from build123d import *

# Parameters (mm, degrees)
BOSS_EXTRUDE1_DEPTH      = 18
BOSS_EXTRUDE1_DEPTH_BACK = 12.815459
SKETCH1_W                = 72.5
SKETCH1_H                = 96.828401578
SHELL1_T                 = 2
SKETCH2_R                = 7.5
CUT_EXTRUDE1_DEPTH       = 2
CHAMFER1_SIZE            = 1
SKETCH5_R                = 5.5
CUT_EXTRUDE2_DEPTH       = 2
CHAMFER2_SIZE            = 1
SKETCH8_W                = 72.5
SKETCH8_H                = 96.828401578
CUT_EXTRUDE5_DEPTH       = 8
BOSS_EXTRUDE3_START      = 10
SKETCH10_W               = 70.5
SKETCH10_H               = 94.828401578
SKETCH10_W_2             = 68.5
SKETCH10_H_2             = 92.828401578
BOSS_EXTRUDE3_DEPTH      = 2
CUT_EXTRUDE6_REACH       = 183.831
SKETCH12_R               = 1.6
FILLET1_R                = 2
BOSS_EXTRUDE4_START      = 10
SKETCH13_R               = 1.65
BOSS_EXTRUDE4_DEPTH      = 2
SKETCH16_R               = 1.65
BOSS_EXTRUDE5_DEPTH      = 2
SKETCH17_R               = 1.65
CUT_EXTRUDE8_DEPTH       = 12.81545914
SKETCH19_W               = 44.967113154
SKETCH19_H               = 24.357186292
BOSS_EXTRUDE6_DEPTH      = 12
CUT_EXTRUDE9_START       = -10.815459
SKETCH18_R               = 3
CUT_EXTRUDE9_DEPTH       = 14
SKETCH14_R               = 1.599946
CUT_EXTRUDE7_DEPTH       = 2


with BuildPart() as part:
    # Sketch1 → Boss-Extrude1 (new, two sides: drawn at the far end of the back side and taken through both)
    with BuildSketch(Plane(origin=(0, 0, 0), x_dir=(1, 0, 0), z_dir=(0, 1, 0)).offset(-BOSS_EXTRUDE1_DEPTH_BACK)):
        with Locations((117.12025684, -15.018542133)):
            Rectangle(SKETCH1_W, SKETCH1_H)
    extrude(amount=BOSS_EXTRUDE1_DEPTH + BOSS_EXTRUDE1_DEPTH_BACK)

    # Shell1 (no face opened: a closed hollow body)
    add(offset(amount=-SHELL1_T, mode=Mode.PRIVATE), mode=Mode.SUBTRACT)

    # Sketch2 → Cut-Extrude1 (cut)
    with BuildSketch(Plane(origin=(0, 0, -33.395658656), x_dir=(-1, 0, 0), z_dir=(0, 0, -1))):
        with Locations((-114.89374317, -0.00045914)):
            Circle(SKETCH2_R)
    extrude(amount=-CUT_EXTRUDE1_DEPTH, mode=Mode.SUBTRACT)

    # Chamfer1
    chamfer1_edges = [part.edges().sort_by_distance(p)[0] for p in [
        (122.39374317, -0.00045914, -33.395658656),
    ]]
    chamfer(chamfer1_edges, length=CHAMFER1_SIZE)

    # Sketch5 → Cut-Extrude2 (cut)
    with BuildSketch(Plane.XY.offset(63.432742922)):
        with Locations((100.762134065, -2.34045914)):
            Circle(SKETCH5_R)
    extrude(amount=-CUT_EXTRUDE2_DEPTH, mode=Mode.SUBTRACT)

    # Chamfer2
    chamfer2_edges = [part.edges().sort_by_distance(p)[0] for p in [
        (95.262134065, -2.34045914, 63.432742922),
    ]]
    chamfer(chamfer2_edges, length=CHAMFER2_SIZE)

    # Sketch8 → Cut-Extrude5 (cut)
    with BuildSketch(Plane(origin=(0, 18, 0), x_dir=(1, 0, 0), z_dir=(0, 1, 0))):
        with Locations((117.12025684, -15.018542133)):
            Rectangle(SKETCH8_W, SKETCH8_H)
    extrude(amount=-CUT_EXTRUDE5_DEPTH, mode=Mode.SUBTRACT)

    # Sketch10 → Boss-Extrude3 (add)
    with BuildSketch(Plane(origin=(0, 0, 0), x_dir=(1, 0, 0), z_dir=(0, 1, 0)).offset(BOSS_EXTRUDE3_START)):
        with Locations((117.12025684, -15.018542133)):
            Rectangle(SKETCH10_W, SKETCH10_H)
        with Locations((117.12025684, -15.018542133)):
            Rectangle(SKETCH10_W_2, SKETCH10_H_2, mode=Mode.SUBTRACT)
    extrude(amount=BOSS_EXTRUDE3_DEPTH)

    # Sketch12 → Cut-Extrude6 (cut, up to next)
    with BuildSketch(Plane.XY.offset(63.432742922), mode=Mode.PRIVATE) as cut_extrude6_sk1:
        with Locations((109.796270245, -4.680244976)):
            Circle(SKETCH12_R)
    cut_extrude6_tool1 = extrude(cut_extrude6_sk1.sketch, amount=-CUT_EXTRUDE6_REACH, mode=Mode.PRIVATE) & part.part
    add(cut_extrude6_tool1.solids().sort_by_distance((109.79627, -4.680245, 63.432743))[0], mode=Mode.SUBTRACT)

    # Fillet1
    fillet1_edges = [part.edges().sort_by_distance(p)[0] for p in [
        (80.87025684, -1.4077295, -33.395658656),
        (153.37025684, -1.4077295, -33.395658656),
        (153.37025684, -1.4077295, 63.432742922),
        (80.87025684, -1.4077295, 63.432742922),
    ]]
    fillet(fillet1_edges, radius=FILLET1_R)

    # Sketch13 → Boss-Extrude4 (add)
    with BuildSketch(Plane(origin=(0, 0, 0), x_dir=(1, 0, 0), z_dir=(0, 1, 0)).offset(BOSS_EXTRUDE4_START)):
        with BuildLine():
            Line((111.12025684, -63.432742922), (123.12025684, -63.432742922))
            ThreePointArc((123.12025684, -63.432742922), (117.12025684, -69.432742922), (111.12025684, -63.432742922))
        make_face()
        with Locations(Location((117.12025684, -66.432742922, 0), (0, 0, 270))):
            Circle(SKETCH13_R, mode=Mode.SUBTRACT)
    boss_extrude4 = extrude(amount=-BOSS_EXTRUDE4_DEPTH)

    # Sketch16 → Boss-Extrude5 (add)
    with BuildSketch(Plane(origin=(0, 10, 0), x_dir=(1, 0, 0), z_dir=(0, 1, 0))):
        with BuildLine():
            Line((111.12025684, 33.395658656), (123.12025684, 33.395658656))
            ThreePointArc((123.12025684, 33.395658656), (117.12025684, 39.395658656), (111.12025684, 33.395658656))
        make_face()
        with Locations(Location((117.12025684, 36.395658656, 0), (0, 0, 270))):
            Circle(SKETCH16_R, mode=Mode.SUBTRACT)
    extrude(amount=-BOSS_EXTRUDE5_DEPTH)

    # Sketch17 → Cut-Extrude8 (cut)
    with BuildSketch(Plane(origin=(0, 0, 0), x_dir=(1, 0, 0), z_dir=(0, 1, 0))):
        with Locations(Location((137.785174065, -38.462742922, 0), (0, 0, 90))):
            Circle(SKETCH17_R)
        with Locations(Location((89.525174065, -37.192742922, 0), (0, 0, 90))):
            Circle(SKETCH17_R)
    extrude(amount=-CUT_EXTRUDE8_DEPTH, mode=Mode.SUBTRACT)

    # Sketch19 → Boss-Extrude6 (add)
    with BuildSketch(Plane.XZ.offset(12.81545914)):
        with Locations((117.12025684, 15.018542133)):
            Rectangle(SKETCH19_W, SKETCH19_H)
    extrude(amount=BOSS_EXTRUDE6_DEPTH)

    # Sketch18 → Cut-Extrude9 (cut)
    with BuildSketch(Plane(origin=(0, 0, 0), x_dir=(1, 0, 0), z_dir=(0, 1, 0)).offset(CUT_EXTRUDE9_START)):
        with Locations(Location((124.62025684, -15.018542133, 0), (0, 0, 270))):
            Circle(SKETCH18_R)
        with Locations(Location((109.62025684, -15.018542133, 0), (0, 0, 270))):
            Circle(SKETCH18_R)
    extrude(amount=-CUT_EXTRUDE9_DEPTH, mode=Mode.SUBTRACT)

    # Mirror1: Boss-Extrude4 across plane
    add(boss_extrude4.mirror(Plane.XY.offset(15.018542133)))

    # Sketch14 → Cut-Extrude7 (cut)
    with BuildSketch(Plane(origin=(0, -10.81545914, 0), x_dir=(1, 0, 0), z_dir=(0, 1, 0))):
        with Locations(Location((140.517827737, -46.462742922, 0), (0, 0, 270))):
            Circle(SKETCH14_R)
        with Locations(Location((92.257827737, -45.192742922, 0), (0, 0, 270))):
            Circle(SKETCH14_R)
    extrude(amount=-CUT_EXTRUDE7_DEPTH, mode=Mode.SUBTRACT)


solid = part.part
CAD build for the part. Positions are in the model's coordinates, mm. A direction names the side the tool comes from. Coordinates: 2 decimals unless noted, no trailing zeros. Order: outer loops, then holes, each group sorted by start corner. A loop starts at its lowest first (then second) coordinate and runs counter-clockwise, first axis right, second up.
Item 1: Band-saw the part on B-B on z = 29. List the corners of the cut face in (x, y).
Check sheet entries:
outline: (80.87, -12.82) - (153.37, -12.82) - (153.37, 10) - (152.37, 10) - (152.37, 12) - (151.37, 12) - (151.37, -10.82) - (82.87, -10.82) - (82.87, 12) - (81.87, 12) - (81.87, 10) - (80.87, 10) - close
Item 2: Two-plate mould, pull along X, no slides. Class faces 1 (the face through (117, 8, 64)), 2 (the face through (80.87, -2, 16)), 3 (the face through (117, 0, 61.433)): +X half, -X half, draft (parallel to the pull), parting line (faces both ways), or undercut.
Check sheet entries:
face 1: draft
face 2: -X half
face 3: undercut
Item 3: Band-saw the part on A-A on x = 144.5. List the corners of the cut face in (y, z), plus the area to 3 significant figures.
Check sheet entries:
outline: (-12.82, -33.4) - (10, -33.4) - (10, -32.4) - (12, -32.4) - (12, -31.4) - (-10.82, -31.4) - (-10.82, 61.43) - (12, 61.43) - (12, 62.43) - (10, 62.43) - (10, 63.43) - (-12.82, 63.43) - close
area: 281 mm2
Item 4: Pin check, flat tips, straight feed: pin 1 Ø1.5 at (x, z) = (132.5, -10.5) entering from +Y; pin 2 Ø10 at (x, y) = (94.5, 1.5) entering from -Z; pin 3 Ø5 at (x, z) = (126.5, 17) entering from -Y; pin 4 Ø1.6 at (y, z) = (11, -6) entering from +X. Stop position of each tip, or through.
Check sheet entries:
pin 1: stops at y = -10.82
pin 2: stops at z = -33.4
pin 3: stops at y = -24.82
pin 4: stops at x = 152.37
Item 5: Band-saw the part on C-C on y = -18. List the corners of the cut face in (x, z).
Check sheet entries:
outline: (94.64, 2.84) - (139.6, 2.84) - (139.6, 27.2) - (94.64, 27.2) - close; hole circle Ø6 at (109.62, 15.02); hole circle Ø6 at (124.62, 15.02)
Item 6: 3-axis set-ups, long thin cutter, end or side, ignore diameter. For faces 4 (the face through (108.2, -4.6, 62.4)), 5 (the face through (136.15, -11.8, 38.68)), 6 (the face through (151.37, 0, 16)), 7 (the face through (117, -19, 27.197)): which of +Z, -Z, +X, -X, +Y, -Y reach the whole face in a straight line?
Check sheet entries:
face 4: +Z
face 5: +Y, -Y
face 6: +Y
face 7: +Z, +X, -X, -Y
Item 7: Drill centre lines: L1, parallel to X at y = -4, z = 39.5; L2, parallel to Z at x = 150.5, y = -7; L3, parallel to X at y = 10.5, z = -8.5. Where is each one in solid material? Low to high.
Check sheet entries:
L1: x = 80.87 to 82.87, 151.37 to 153.37
L2: z = -33.4 to -31.4, 61.43 to 63.43
L3: x = 81.87 to 82.87, 151.37 to 152.37
